Part model, mm, in its own coordinate system. Face numbers are marked on the shaded views. A direction names the side the tool comes from. Give positions to 0.01 mm unless a question says otherwise; leave off trailing zeros. Order: outer loops, then holes, each group sorted by start corner. A loop starts at its lowest first (then second) coordinate and runs counter-clockwise, first axis right, second up.
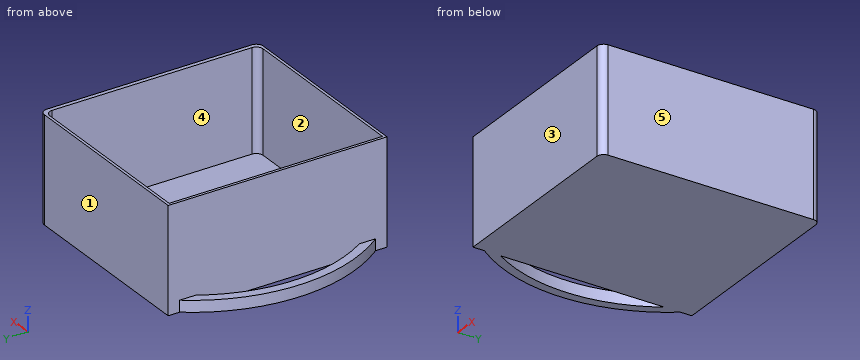
from build123d import *

# Parameters (mm, degrees)
SKETCH_1_W          = 86
SKETCH_1_H          = 95.9
EXTRUDE_1_DEPTH     = 46.1
EXTRUDE_2_DEPTH     = 5
SKETCH_3_W          = 83
SKETCH_3_H          = 93.5
CUT_EXTRUDE_1_DEPTH = 44.5
FILLET_1_R          = 3


with BuildPart() as part:
    # Эскиз1 → Бобышка-Вытянуть1 (new body)
    with BuildSketch(Plane.XY):
        Rectangle(SKETCH_1_W, SKETCH_1_H)
    extrude(amount=EXTRUDE_1_DEPTH)

    # Эскиз2 → Бобышка-Вытянуть2 (add)
    with BuildSketch(Plane.XY):
        with BuildLine():
            Line((-43, 42.95), (-43, 35.870635623))
            ThreePointArc((-43, 35.870635623), (-53.275135929, 0), (-43, -35.870635623))
            Line((-43, -35.870635623), (-43, -42.95))
            ThreePointArc((-43, -42.95), (-57.275135929, 0), (-43, 42.95))
        make_face()
    extrude(amount=EXTRUDE_2_DEPTH)

    # Эскиз3 → Вырез-Вытянуть1 (cut)
    with BuildSketch(Plane.XY.offset(46.1)):
        with Locations((-0.3, 0)):
            Rectangle(SKETCH_3_W, SKETCH_3_H)
    extrude(amount=-CUT_EXTRUDE_1_DEPTH, mode=Mode.SUBTRACT)

    # Скругление1
    fillet_1_edges = [part.edges().sort_by_distance(p)[0] for p in [
        (41.2, 46.75, 23.85),
        (41.2, -46.75, 23.85),
        (43, 47.95, 23.05),
        (43, -47.95, 23.05),
    ]]
    fillet(fillet_1_edges, radius=FILLET_1_R)


solid = part.part
Item 1: Drill centre lines: probe 1 along X at (y, z) = (-32, 17); probe 2 along Y at (x, z) = (-11, 33.5); probe 3 along Z at (x, y) = (-15.5, -33). Where is each one in solid material? Low to high.
Item 2: Band-saw the part on A-A on z = 29.5. List the corners of the cut face in (x, y).
Item 3: Band-saw the part on D-D on y = -8. List the corners of the cut face in (x, z).
Item 4: Band-saw the part on B-B on y = -21. List the corners of the cut face in (x, z), plus the area to 3 significant figures.
Item 5: Band-saw the part on C-C on x = 0. List the corners of the cut face in (y, z).
Item 6: Pull direction X, two halves, no side cores. Call the marked faces 3, 4 and 5: released by +X, released by -X, zero draft, split by the parting line, or undercut.
Item 7: Drop flat-ended pins along their axis: P1, Ø1.5, axis at x = -25, y = -2, coming from the +Z side; P2, Ø4.5, axis at x = -53, y = -3.5, coming from the +Z side; P3, Ø3, axis at y = -24, z = 23.5, coming from the -X side. Give the stop position or say it passes through.
Item 8: Which spindle directions (+Z, -Z, +X, -X, +Y, -Y) get a long thin tool onto all of the face, cutting with end or side? Do the marked faces 1 and 2. Say none if no direction does.
Working result:
1. probe 1: x = -43 to -41.8, 41.2 to 43
1. probe 2: y = -47.95 to -46.75, 46.75 to 47.95
1. probe 3: z = 0 to 1.6
2. outline: (-43, -47.95) - (40, -47.95) arc R3 ccw to (43, -44.95) - (43, 44.95) arc R3 ccw to (40, 47.95) - (-43, 47.95) - close; hole (-41.8, -46.75) - (38.2, -46.75) arc R3 ccw to (41.2, -43.75) - (41.2, 43.75) arc R3 ccw to (38.2, 46.75) - (-41.8, 46.75) - close
3. outline: (-56.83, 0) - (-52.8, 0) - (-52.8, 5) - (-56.83, 5) - close; (-43, 0) - (43, 0) - (43, 46.1) - (41.2, 46.1) - (41.2, 1.6) - (-41.8, 1.6) - (-41.8, 46.1) - (-43, 46.1) - close
4. outline: (-54.13, 0) - (-49.94, 0) - (-49.94, 5) - (-54.13, 5) - close; (-43, 0) - (43, 0) - (43, 46.1) - (41.2, 46.1) - (41.2, 1.6) - (-41.8, 1.6) - (-41.8, 46.1) - (-43, 46.1) - close
4. area: 292 mm2
5. outline: (-47.95, 0) - (47.95, 0) - (47.95, 46.1) - (46.75, 46.1) - (46.75, 1.6) - (-46.75, 1.6) - (-46.75, 46.1) - (-47.95, 46.1) - close
6. face 3: zero draft
6. face 4: undercut
6. face 5: released by +X
7. P1: stops at z = 1.6
7. P2: stops at z = 5
7. P3: stops at x = -43
8. face 1: +Z, -Z, +X, -X, +Y
8. face 2: +Z
